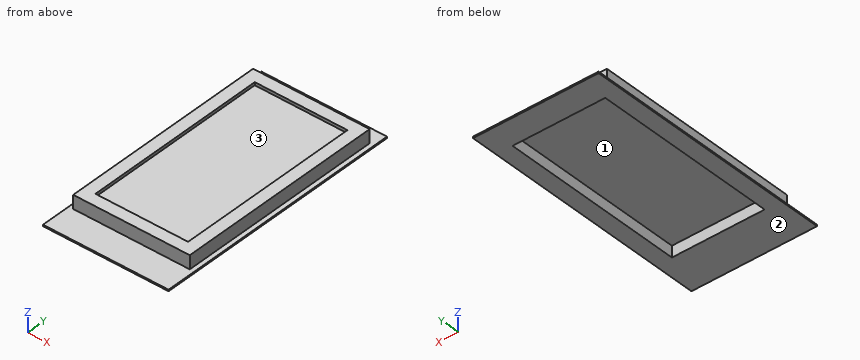
```python
from build123d import *

# Parameters (mm, degrees)
F0_W     = 780
F0_H     = 1400
F0_W_2   = 620
F0_H_2   = 1240
F1_DEPTH = 100
F2_W     = 840
F2_H     = 1700
F2_W_2   = 780
F2_H_2   = 1400
F3_DEPTH = 10
F5_W     = 620
F5_H     = 1240
F6_DEPTH = 5


with BuildPart() as f1:
    # F0 (on Top) → F1 (new body)
    with BuildSketch(Plane.XY):
        with Locations((390, 700)):
            Rectangle(F0_W, F0_H)
        with Locations((390, 700)):
            Rectangle(F0_W_2, F0_H_2, mode=Mode.SUBTRACT)
    extrude(amount=F1_DEPTH)

    # F2 (on face) → F3 (join)
    with BuildSketch(Plane(origin=(0, 0, 0), x_dir=(1, 0, 0), z_dir=(0, 0, -1))):
        with Locations((390, -650)):
            Rectangle(F2_W, F2_H)
        with Locations((390, -700)):
            Rectangle(F2_W_2, F2_H_2, mode=Mode.SUBTRACT)
    extrude(amount=-F3_DEPTH)

    # F5 (on offset) → F6 (join)
    with BuildSketch(Plane.XY.offset(75)):
        with Locations((390, 700)):
            Rectangle(F5_W, F5_H)
    extrude(amount=F6_DEPTH)


solid = f1.part
```
CAD build for the part. Positions are in the model's coordinates, mm. Face numbers are marked on the shaded views. Round coordinates to 2 decimals unless told otherwise and drop trailing zeros. Loops run counter-clockwise (first coordinate to the right, second up) from the corner with the lowest first, then second, coordinate; pieces in that order, holes last. Notation, with made-up numbers: M 40.25,38 L 92.25,38 A29 ccw 92.25,61 Z; hole C 12.5,-13.5 d4. An arc over 180 degrees is marked long. Return JSON: item names as keys, results as strings. Group by question number.
(1) Saw through at B-B, the plane x = 439. List the corners of the cut face in (y, z), and give its area (3 significant figures).
(2) Saw through at C-C, the plane y = 459. List the corners of the cut face in (x, z), and give its area (3 significant figures).
(3) Drop flat-ended pins along their axis: P1, Ø4, axis at y = 500.5, z = 83.5, coming from the +X side; P2, Ø6, axis at x = 202, y = 1269.5, coming from the -Z side; P3, Ø5, axis at y = 1283.5, z = 55.5, coming from the -X side. Give the stop position or say it passes through.
(4) Saw through at A-A, the plane z = 28. List the corners of the cut face in (x, y), and give its area (3 significant figures).
(5) Mould opens along X. For the marked faces 1, 2 and 3 say: +X half, -X half, draft (parallel to the pull), parting line (faces both ways), or undercut.
(6) Wall check: probe 1 along X at (y, z) = (1026, 46.5); probe 2 along Y at (x, z) = (678.5, 60.5); probe 3 along X at (y, z) = (1168.5, 9). Give the ranges that are in metal, low to high. Write a range as [from, to].
(7) Saw through at D-D, the plane x = 744.5. List the corners of the cut face in (y, z).
Answer list:
{
 "1": {"outline": "M -200,0 L 80,0 L 80,75 L 1320,75 L 1320,0 L 1500,0 L 1500,10 L 1400,10 L 1400,100 L 1320,100 L 1320,80 L 80,80 L 80,100 L 0,100 L 0,10 L -200,10 Z", "area": "25,200 mm2"},
 "2": {"outline": "M -30,0 L 80,0 L 80,75 L 700,75 L 700,0 L 810,0 L 810,10 L 780,10 L 780,100 L 700,100 L 700,80 L 80,80 L 80,100 L 0,100 L 0,10 L -30,10 Z", "area": "19,700 mm2"},
 "3": {"P1": "x = 780", "P2": "z = 75", "P3": "x = 0"},
 "4": {"outline": "M 0,0 L 780,0 L 780,1400 L 0,1400 Z; hole M 80,80 L 700,80 L 700,1320 L 80,1320 Z", "area": "323,000 mm2"},
 "5": {"face 1": "undercut", "face 2": "draft", "face 3": "undercut"},
 "6": {"probe 1": "[0, 80], [700, 780]", "probe 2": "[0, 80], [1320, 1400]", "probe 3": "[-30, 80], [700, 810]"},
 "7": {"outline": "M -200,0 L 1500,0 L 1500,10 L 1400,10 L 1400,100 L 0,100 L 0,10 L -200,10 Z"}
}
